Verification items for the finished model (mm, model axes). Face numbers are marked on the shaded views. A direction names the side the tool comes from. Coordinates: 2 decimals unless noted, no trailing zeros. Order: outer loops, then holes, each group sorted by start corner. A loop starts at its lowest first (then second) coordinate and runs counter-clockwise, first axis right, second up. Notation, with made-up numbers: (1.25, 82) -> (25.25, 82) arc R14 cw to (25.25, 107) -> close; hole circle Ø11 at (62, -29.5). An arc over 180 degrees is marked (long way). Write each question's results on one line, items separated by ' | '. Start each with the question number.
(1) Cross-section at B-B on x = 4. Enter the section's corners in (y, z) (1 decimal).
(2) Cross-section at C-C on y = -4.25. Enter the section's corners in (x, z), and give its area (3 significant figures).
(3) Set-up check for the marked faces 1, 2 and 3: record each of +Z, -Z, +X, -X, +Y, -Y from which the full face is reachable in a straight line by a thin tool's end or side.
(4) Thickness scan on probe 1 along Z at (x, y) = (-9.5, 4); probe 2 along Y at (x, z) = (-0.25, 1.3) (3 decimals); probe 3 along X at (y, z) = (1, 1.5). Record the ranges inside material, lowest first. Write a range as [from, to].
(5) Go/stop test with flat-tipped pins: pin 1 (0.8 mm diameter, centred on x = 1, z = 1, fed in from -Y); pin 2 (1.2 mm diameter, centred on x = 0, y = -10.5, fed in from +Z); pin 3 (0.8 mm diameter, centred on x = -2.5, z = 1, fed in from +Y). Record where each tip stops, or that it passes through.
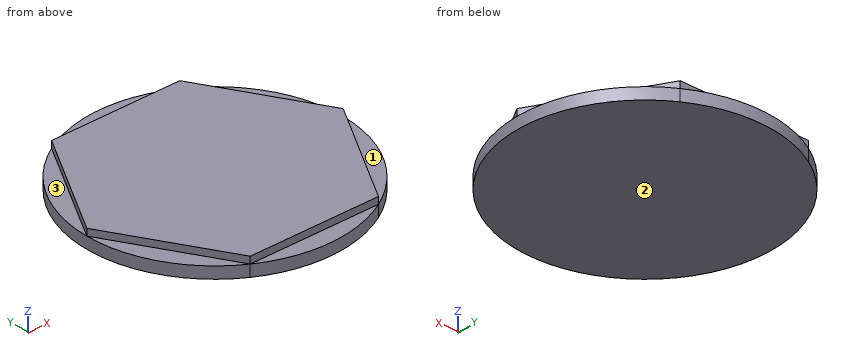
Solid Edge part; units mm, degrees
sketch "Sketch1" plane through (0, 0, 0) normal (0, 0, 1) x (1, 0, 0)
  line L0 (5.4993, -9.525) -> (10.9985, 0)
  line L1 (10.9985, 0) -> (5.4993, 9.525)
  line L2 (5.4993, 9.525) -> (-5.4993, 9.525)
  line L3 (-5.4993, 9.525) -> (-10.9985, 0)
  line L4 (-10.9985, 0) -> (-5.4993, -9.525)
  line L5 (-5.4993, -9.525) -> (5.4993, -9.525)
extrude "Protrusion1" add sketch "Sketch1" along normal blind 1.5875
sketch "Sketch2" plane through (0, 0, 0) normal (0, 0, 1) x (1, 0, 0)
  circle A0 centre (0, 0) radius 10.9985
extrude "ExtrudedCutout_1" add sketch "Sketch2" along normal blind 1
Results are:
1) outline: (-10.2, 0) -> (10.2, 0) -> (10.2, 1) -> (9.5, 1) -> (9.5, 1.6) -> (-9.5, 1.6) -> (-9.5, 1) -> (-10.2, 1) -> close
2) outline: (-10.14, 0) -> (10.14, 0) -> (10.14, 1) -> (8.54, 1) -> (8.54, 1.59) -> (-8.54, 1.59) -> (-8.54, 1) -> (-10.14, 1) -> close | area: 30.3 mm2
3) face 1: +Z, +X, -Y | face 2: -Z, +X, -X, +Y, -Y | face 3: +Z, -X, +Y
4) probe 1: z = [0, 1] | probe 2: y = [-9.525, 9.525] | probe 3: x = [-10.42, 10.42]
5) pin 1: stops at y = -10.98 | pin 2: stops at z = 1 | pin 3: stops at y = 10.8
